Autodesk Inventor part; units mm, degrees
ref_plane "YZ Plane" through (0, 0, 0) normal (1, 0, 0) x (0, 1, 0)
ref_plane "XZ Plane" through (0, 0, 0) normal (0, 1, 0) x (-1, 0, 0)
ref_plane "XY Plane" through (0, 0, 0) normal (0, 0, 1) x (1, 0, 0)
sketch "Sketch1" plane through (0, 0, 0) normal (0, 1, 0) x (-1, 0, 0)
  arc A0 (0, -35.5) -> (0, 35.5) centre (0, 0) ccw construction
  arc A1 (-2.5809, -40.3369) -> (-17.4082, 36.0494) centre (1.0497, 0) ccw construction
  arc A2 (39.0973, -13.8791) -> (40.8076, 7.7173) centre (1.0497, 0) ccw construction
  line L0 (41.5497, -0.0049) -> (41.3517, -4) construction
  line L1 (41.5497, -0.0049) -> (41.3527, 3.9902) construction
  arc A3 (41.3517, -4) -> (41.3527, 3.9902) centre (1.0497, 0) ccw
  line L2 (35.5, 0) -> (35.5, -4) construction
  line L3 (35.5, 0) -> (35.5, 4) construction
  arc A4 (35.2739, -4) -> (35.275, 3.9902) centre (0, 0) ccw construction
  arc A5 (35.2739, -4) -> (35.275, 3.9902) centre (0, 0) ccw
  line L4 (41.3527, 3.9902) -> (35.275, 3.9902)
  line L5 (41.3517, -4) -> (35.2739, -4)
  dimension "d7" = 0
  dimension "d8" = 40.5
  dimension "d9" = 35.5
  dimension "d14" = 4
  dimension "d15" = 4
  dimension "d18" = 4
  dimension "d19" = 4
extrude "Extrusion1" add sketch "Sketch1" along normal blind 3
sketch "Sketch2" plane through (0, 3, 0) normal (0, 1, 0) x (1, 0, 0)
  arc A0 (-41.3517, 4) -> (-41.3527, -3.9902) centre (-1.0497, 0) ccw
  line L0 (-41.3527, -3.9902) -> (-35.275, -3.9902)
  arc A1 (-35.2739, 4) -> (-35.275, -3.9902) centre (0, 0) ccw
  line L1 (-35.2739, 4) -> (-41.3517, 4)
  circle A2 centre (-38.3128, 0) radius 1.75
  point P0 (0, 0)
  dimension "d22" = 3.5
extrude "Extrusion2" cut sketch "Sketch2" along normal through all both and the other way through all contours A2
fillet "Fillet1" radius 1 4 edges at (-41.3527, 1.5, 3.9902) (-41.3517, 1.5, -4) (-35.2739, 1.5, -4) (-35.275, 1.5, 3.9902)
properties part number "reverse gear link block"
The listing builds one solid part. Answer for the finished solid, in the listing's coordinates (mm). Give positions to 0.01 mm unless a question says otherwise; leave off trailing zeros. Order: outer loops, then holes, each group sorted by start corner. A loop starts at its lowest first (then second) coordinate and runs counter-clockwise, first axis right, second up. Notation, with made-up numbers: (-21, -37) - (28, -37) arc R23 ccw to (28, -3) - close; hole circle Ø5 at (8, 48.5). An arc over 180 degrees is marked (long way). Answer in a Markdown table with one row per item. Add a question column.
Q1. Find the intervals of material crossed by line 1 along X through (y, z) = (1.05, 0); line 2 along Z through (x, y) = (-38.25, 2); line 3 along Z through (x, y) = (-37.25, 2.7), in increasing order. Write a range as [from, to].
Q2. The part is cut by section A-A (z = 0). Determine the outline of the cut face in (x, y), then the cut area to 3 significant figures.
Q3. The part is cut by section C-C (y = 1.6). Determine the outline of the cut face in (x, z), then the cut area to 3 significant figures.
Q4. The part is cut by section B-B (x = -38.5). Determine the outline of the cut face in (y, z).
Q5. Given P1, Ø1, axis at y = 2.5, z = 2, coming from the +X side; P2, Ø2, axis at x = -38.31, z = 0, coming from the -Y side, each flat-ended and moving along its own axis, determine where each tip first touches the part or whether it passes through.
Determined:
| question | item | result |
|---|---|---|
| 1 | line 1 | x = [-41.55, -40.06], [-36.56, -35.5] |
| 1 | line 2 | z = [-4, -1.75], [1.75, 3.99] |
| 1 | line 3 | z = [-4, -1.39], [1.39, 3.99] |
| 2 | outline | (-41.55, 0) - (-40.06, 0) - (-40.06, 3) - (-41.55, 3) - close; (-36.56, 0) - (-35.5, 0) - (-35.5, 3) - (-36.56, 3) - close |
| 2 | area | 7.65 mm² |
| 3 | outline | (-41.43, -3.08) arc R1 ccw to (-40.44, -4) - (-36.38, -4) arc R1 ccw to (-35.38, -2.92) arc R35.5 cw to (-35.38, 2.91) arc R1 ccw to (-36.38, 3.99) - (-40.44, 3.99) arc R1 ccw to (-41.43, 3.07) arc R40.5 ccw to start; hole circle Ø3.5 at (-38.31, 0) |
| 3 | area | 37.9 mm² |
| 4 | outline | (0, -4) - (3, -4) - (3, -1.74) - (0, -1.74) - close; (0, 1.74) - (3, 1.74) - (3, 3.99) - (0, 3.99) - close |
| 5 | P1 | stops at x = -35.41 |
| 5 | P2 | passes through |
